from build123d import *

# Parameters (mm, degrees)
F0_R     = 5.5
F0_R_2   = 20
F1_DEPTH = 10


with BuildPart() as f1:
    # F0 (on Top) → F1 (new body)
    with BuildSketch(Plane.XY):
        with BuildLine():
            ThreePointArc((0, 30), (8.786797, 8.786797), (30, 0))
            Line((30, 0), (153, 0))
            ThreePointArc((153, 0), (174.213203, 8.786797), (183, 30))
            ThreePointArc((183, 30), (174.213203, 51.213203), (153, 60))
            Line((153, 60), (30, 60))
            ThreePointArc((30, 60), (8.786797, 51.213203), (0, 30))
        make_face()
        with Locations((20, 30)):
            Circle(F0_R, mode=Mode.SUBTRACT)
        with Locations((91.5, 30)):
            Circle(F0_R_2, mode=Mode.SUBTRACT)
        with Locations((163, 30)):
            Circle(F0_R, mode=Mode.SUBTRACT)
    extrude(amount=F1_DEPTH)


solid = f1.part
The model under review builds one solid part; all positions refer to its coordinate system, in mm. Coordinates: 2 decimals unless noted, no trailing zeros. Write each loop counter-clockwise with the first axis right and the second up, starting at its lowest first coordinate (ties: lowest second). Pieces come first, ordered by that corner, then holes. Notation, with made-up numbers: M 62,-0.5 L 85,-0.5 A5 cw 85,7.5 Z; hole C 44,40.25 d9. An arc over 180 degrees is marked long. Put each result on its own line as item: value.
1) Add section C-C on y = 14. Give the boundary of the cut face in (x, z), then the cut area to 3 significant figures.
Computed:
outline: M 4.62,0 L 79.5,0 L 79.5,10 L 4.62,10 Z; M 103.5,0 L 178.38,0 L 178.38,10 L 103.5,10 Z
area: 1,500 mm2
2) Draft analysis for pull direction Y (two halves, no side actions). For faces 1 (the cylindrical face through (71.52, 30.88, 4.93)), 2 (the flat face through (90.2, 50.4, 0)), 3 (the flat face through (92, 60, 5)), state which applies: released by +Y, released by -Y, zero draft, split by the parting line, or undercut.
Computed:
face 1: undercut
face 2: zero draft
face 3: released by +Y
3) Clearance check with flat-ended pins moving along their axes: pin 1 Ø6 at (y, z) = (29, 8) entering from -X; pin 2 Ø1.5 at (y, z) = (20.5, 4) entering from -X; pin 3 Ø1 at (y, z) = (46.5, 7) entering from -X. State where each tip first meets the part, or that it passes through.
Computed:
pin 1: stops at x = 0
pin 2: stops at x = 1.3
pin 3: stops at x = 4.62
4) Add section A-A on z = 3.5. Give the boundary of the cut face in (x, y).
Computed:
outline: M 0,30 A30 ccw 30,0 L 153,0 A30 ccw 183,30 A30 ccw 153,60 L 30,60 A30 ccw Z; hole C 20,30 d11; hole C 91.5,30 d40; hole C 163,30 d11
5) Wall thickness on probe 1 along X at (y, z) = (28, 7); probe 2 along Y at (x, z) = (92, 7.75); probe 3 along X at (y, z) = (25, 3): over which ranges is each line inside the solid? List them lowest first. Write a range as [from, to].
Computed:
probe 1: x = [0.07, 14.88], [25.12, 71.6], [111.4, 157.88], [168.12, 182.93]
probe 2: y = [0, 10.01], [49.99, 60]
probe 3: x = [0.42, 17.71], [22.29, 72.14], [110.86, 160.71], [165.29, 182.58]
6) Add section D-D on y = 32. Give the boundary of the cut face in (x, z).
Computed:
outline: M 0.07,0 L 14.88,0 L 14.88,10 L 0.07,10 Z; M 25.12,0 L 71.6,0 L 71.6,10 L 25.12,10 Z; M 111.4,0 L 157.88,0 L 157.88,10 L 111.4,10 Z; M 168.12,0 L 182.93,0 L 182.93,10 L 168.12,10 Z
7) Add section B-B on x = 86.5. Give the boundary of the cut face in (y, z), then the cut area to 3 significant figures.
Computed:
outline: M 0,0 L 10.64,0 L 10.64,10 L 0,10 Z; M 49.36,0 L 60,0 L 60,10 L 49.36,10 Z
area: 213 mm2
